The model under review builds one solid part; all positions refer to its coordinate system, in mm. A direction names the side the tool comes from. Give positions to 0.01 mm unless a question says otherwise; leave off trailing zeros. Order: outer loops, then holes, each group sorted by start corner. A loop starts at its lowest first (then second) coordinate and runs counter-clockwise, first axis right, second up. Notation, with made-up numbers: (11, 84) - (33, 84) arc R10 ccw to (33, 98) - close; hole circle Ø4 at (58.5, 76.25). An arc over 180 degrees is marked (long way). Use a Markdown table: item, result. Add a question column.
Autodesk Inventor part; units mm, degrees
ref_plane "YZ Plane" through (0, 0, 0) normal (1, 0, 0) x (0, 1, 0)
ref_plane "XZ Plane" through (0, 0, 0) normal (0, 1, 0) x (-1, 0, 0)
ref_plane "XY Plane" through (0, 0, 0) normal (0, 0, 1) x (1, 0, 0)
sketch "スケッチ22" plane through (0, 0, 0) normal (0, 0, 1) x (1, 0, 0)
  line L0 (-6.9456, -9.9484) -> (6.9456, -9.9484)
  line L1 (6.9456, -9.9484) -> (6.9456, 9.9484)
  line L2 (6.9456, 9.9484) -> (-6.9456, 9.9484)
  line L3 (-6.9456, 9.9484) -> (-6.9456, -9.9484)
  line L4 (-6.9456, -9.9484) -> (6.9456, 9.9484) construction
  line L5 (6.9456, -9.9484) -> (-6.9456, 9.9484) construction
  point P0 (0, 0)
extrude "押し出し14" add sketch "スケッチ22" along normal blind 5
sketch "スケッチ23" plane through (0, 0, 5) normal (0, 0, 1) x (1, 0, 0)
  line L0 (3.4613, 4.9054) -> (3.4613, -4.9971) construction
  line L1 (2.1075, 4.9054) -> (2.1075, -4.9971)
  line L2 (4.8151, -4.9971) -> (4.8151, 4.9054)
  arc A0 (4.8151, 4.9054) -> (2.1075, 4.9054) centre (3.4613, 4.9054) ccw
  arc A1 (2.1075, -4.9971) -> (4.8151, -4.9971) centre (3.4613, -4.9971) ccw
  point P0 (0, 0)
  point P1 (3.4613, -0.0458)
extrude "押し出し15" cut sketch "スケッチ23" against normal blind 2
properties material "A5052"
Q1. Clearance check with a flat-ended pin moving along its axis: P1, Ø2, axis at x = 3.5, y = -0.5, coming from the +Z side. State where the tip first meets the part, or that it passes through.
Q2. Draft analysis for pull direction Y (two halves, no side actions). For faces 1 (the flat face through (0, -9.948, 2)), 2 (the cylindrical face through (3.43, -6.35, 4.01)), 3 (the flat face through (6.946, 0, 2)), 4 (the flat face through (0, 9.948, 2)), state which applies: pulls with the +Y half, pulls with the -Y half, needs draft (parallel to the pull), parting line crosses it, or undercut.
Q3. We need section B-B (y = -2.25). Write out the cut boundary in (x, z), plus the area to 3 significant figures.
Q4. We need section A-A (z = 4.5). Write out the cut boundary in (x, y), plus the area to 3 significant figures.
Q5. Wall thickness on probe 1 along X at (y, z) = (-4.25, 3.45); probe 2 along Z at (x, y) = (3.25, 3.5); probe 3 along Y at (x, z) = (2.5, 3.35): over which ranges is each line inside the solid? List them lowest first.
Q6. We need section C-C (y = 6). Write out the cut boundary in (x, z).
Q7. Machinability: for faces 5 (the flat face through (2.108, 0, 4)), 6 (the flat face through (0, 0, 0)), which of the approach directions +Z, -Z, +X, -X, +Y, -Y give a long, thin tool a straight path to every point of the face, cutting with its end or side? Answer none if there is none.
Here are the results:
| question | item | result |
|---|---|---|
| 1 | P1 | z = 3 |
| 2 | face 1 | pulls with the -Y half |
| 2 | face 2 | undercut |
| 2 | face 3 | needs draft |
| 2 | face 4 | pulls with the +Y half |
| 3 | outline | (-6.95, 0) - (6.95, 0) - (6.95, 5) - (4.82, 5) - (4.82, 3) - (2.11, 3) - (2.11, 5) - (-6.95, 5) - close |
| 3 | area | 64.0 mm2 |
| 4 | outline | (-6.95, -9.95) - (6.95, -9.95) - (6.95, 9.95) - (-6.95, 9.95) - close; hole (2.11, -5) arc R1.35 ccw to (4.82, -5) - (4.82, 4.91) arc R1.35 ccw to (2.11, 4.91) - close |
| 4 | area | 244 mm2 |
| 5 | probe 1 | -6.95 to 2.11, 4.82 to 6.95 |
| 5 | probe 2 | 0 to 3 |
| 5 | probe 3 | -9.95 to -5.95, 5.86 to 9.95 |
| 6 | outline | (-6.95, 0) - (6.95, 0) - (6.95, 5) - (4.26, 5) - (4.26, 3) - (2.66, 3) - (2.66, 5) - (-6.95, 5) - close |
| 7 | face 5 | +Z |
| 7 | face 6 | -Z, +X, -X, +Y, -Y |
